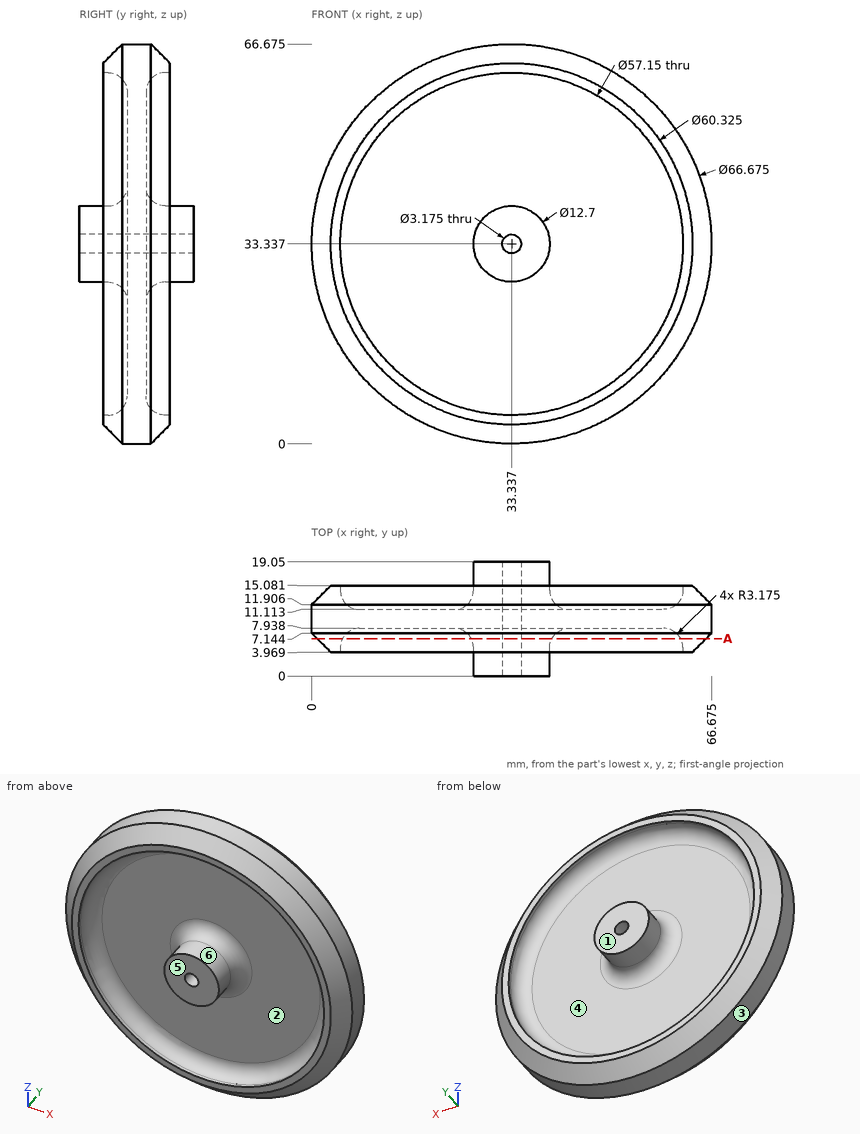
The drawing under review shows one solid part. Ordinate dimensions are in mm from its lowest x, y, z. A direction names the side the tool comes from. Round coordinates to 2 decimals unless told otherwise and drop trailing zeros. One line per question, with ' | ' between items. Start each with the question number.
Item 1: Add section A-A, the plane y = 6.25. Count the separate pieces of the cut face and the enclosed holes in it.
Item 2: Draft analysis for pull direction Z (two halves, no side actions). For the marked faces 1, 2 and 3, state which applies: +Z half, -Z half, draft (parallel to the pull), parting line (faces both ways), or undercut.
Item 3: For pin 1 (4 mm diameter, centred on y = 4.5, z = 29.5, fed in from -X) (1 decimal); pin 2 (8 mm diameter, centred on x = 53, z = 51.5, fed in from -Y); pin 3 (1.5 mm diameter, centred on x = 28, y = 3.5, fed in from -Z) (1 decimal); pin 4 (15 mm diameter, centred on x = 28, z = 26.5, fed in from +Y), all flat-tipped, find the tip position at first contact; note any pin that passes through.
Item 4: Machinability: for the marked faces 4, 5 and 6, which of the approach directions +Z, -Z, +X, -X, +Y, -Y give a long, thin tool a straight path to every point of the face, cutting with its end or side? Answer none if there is none.
Item 5: Wall thickness on line 1 along Y through (x, z) = (51, 40); line 2 along Z through (x, y) = (23, 15) (1 decimal); line 3 along X through (y, z) = (7, 20) (1 decimal): over which ranges is each line inside the solid? List them lowest first. Write a range as [from, to].
Return value:
1) separate pieces: 2 | enclosed holes: 2
2) face 1: draft | face 2: undercut | face 3: parting line
3) pin 1: stops at x = 0.9 | pin 2: stops at y = 3.97 | pin 3: stops at z = 3.4 | pin 4: stops at y = 19.05
4) face 4: +Y | face 5: +Z, -Z, +X, -X, -Y | face 6: -Y
5) line 1: y = [7.94, 11.11] | line 2: z = [4.9, 6.7], [60, 61.8] | line 3: x = [2.9, 9.1], [57.6, 63.7]
